Can you work these out from the model? Positions are in its coordinate system, mm. Face numbers are marked on the shaded views. Give positions to 0.01 mm unless a question says otherwise; leave off trailing zeros. Order: outer loops, then holes, each group sorted by start corner. A loop starts at its lowest first (then second) coordinate and runs counter-clockwise, first axis right, second up.
Item 1: I want a section at B-B, the plane y = 4.75. Write out the boundary of the cut face in (x, z), then the cut area to 3 significant figures.
Item 2: I want a section at D-D, the plane x = -0.75. Write out the boundary of the cut face in (y, z), then the cut area to 3 significant figures.
Item 3: If I drill on line 1 along Z through (x, y) = (-2, 3.9); line 2 along Z through (x, y) = (-2, 2.25); line 3 along X through (y, z) = (8, 4.5), over which ranges is the centre line in solid material (lowest first)?
Item 4: I want a section at C-C, the plane z = -14. Write out the boundary of the cut face in (x, y), then the cut area to 3 significant figures.
Item 5: I want a section at A-A, the plane z = -8. Write out the boundary of the cut face in (x, y).
Item 6: I'm going to push flat-ended pins straight in: pin 1 Ø5 at (x, z) = (-2, -8) entering from -Y; pin 2 Ø1.8 at (x, z) = (-2, -14) entering from -Y; pin 3 Ø3 at (x, z) = (-1, 3.5) entering from -Y. Where does each tip first touch, or does it pass through?
Item 7: If we mould it in two halves opening along X, with no side actions, what happens to the marked faces 1, 2, 3 and 4? For each: +X half, -X half, draft (parallel to the pull), parting line (faces both ways), or undercut.
Autodesk Inventor part; units mm, degrees
ref_plane "YZ Plane" through (0, 0, 0) normal (1, 0, 0) x (0, 1, 0)
ref_plane "XZ Plane" through (0, 0, 0) normal (0, 1, 0) x (-1, 0, 0)
ref_plane "XY Plane" through (0, 0, 0) normal (0, 0, 1) x (1, 0, 0)
sketch "Sketch1" plane through (0, 0, 0) normal (0, 1, 0) x (-1, 0, 0)
  line L0 (-6, 7) -> (10, 7)
  line L1 (10, 7) -> (10, -16)
  line L2 (10, -16) -> (-6, -16)
  line L3 (-6, -16) -> (-6, 7)
  point P0 (0, 0)
  point P1 (2, -8)
  point P2 (2, -14)
  point P3 (2, 4.5)
  dimension "d0" = 16
  dimension "d1" = 23
  dimension "d3" = 8
  dimension "d4" = 2
  dimension "d5" = 20.5
extrude "Extrusion1" add sketch "Sketch1" along normal blind 11.5
hole "Hole1" at (-2, 0, -8) direction (0, 1, 0) diameter 6 end through all
hole "Hole2" at (-2, 0, 4.5) direction (0, 1, 0) diameter 3 end through all
hole "Hole3" at (-2, 0, -14) direction (0, 1, 0) diameter 3 depth 6 tip angle 118
sketch "Sketch3" plane through (6, 0, 7) normal (1, 0, 0) x (0, 0, -1)
  arc A0 (5.6761, 2.9874) -> (5.6761, 5.0126) centre (8.5, 4) ccw
  line L0 (23, 0) -> (0, 0)
  line L1 (23, 0) -> (23, 11.5)
  line L2 (0, 0) -> (0, 11.5)
  line L3 (5.6761, 5.0126) -> (0, 5.0126)
  line L4 (5.6761, 2.9874) -> (0, 2.9874)
  line L5 (0, 5.0126) -> (0, 2.9874)
  point P0 (16, 0)
  point P1 (21, 5.75)
  dimension "d29" = 6
  dimension "d30" = 4
  dimension "d31" = 14.5
  dimension "d32" = 2
  dimension "d33" = 5.75
extrude "Extrusion2" cut sketch "Sketch3" against normal blind 20
hole "Hole4" at (6, 5.75, -14) direction (-1, 0, 0) diameter 3 end through all
thread "Thread1"
thread "Thread2"
thread "Thread3"
thread "Thread4"
properties part number "Chimera Heatblock" material "Aluminum 6061, Welded"
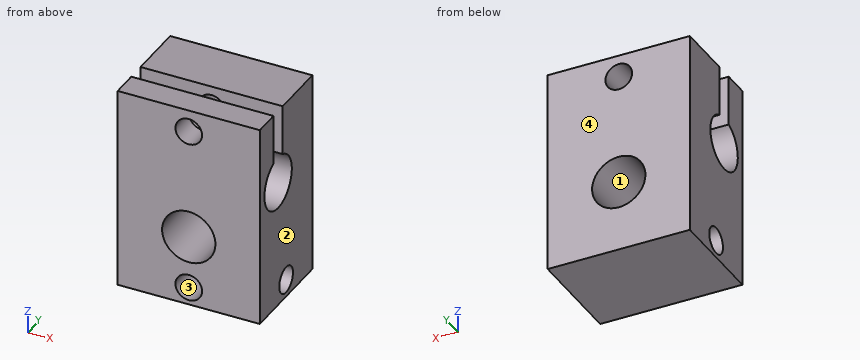
Results list:
1. outline: (-10, -16) - (6, -16) - (6, -15.12) - (-1, -15.12) arc R1.5 cw to (-3, -15.12) - (-10, -15.12) - close; (-10, -12.88) - (-3, -12.88) arc R1.5 cw to (-1, -12.88) - (6, -12.88) - (6, -4.4) - (-10, -4.4) - close; hole circle Ø6 at (-2, -8)
1. area: 120 mm2
2. outline: (0, -16) - (11.5, -16) - (11.5, -10.73) - (0, -10.73) - (0, -13.17) - (4.5, -13.17) arc R1.5 cw (long way) to (4.5, -14.83) - (0, -14.83) - close; (0, -5.27) - (11.5, -5.27) - (11.5, 3.67) - (5.01, 3.67) - (5.01, 1.32) arc R3 cw (long way) to (2.99, 1.32) - (2.99, 3.67) - (0, 3.67) - close; (0, 5.33) - (2.99, 5.33) - (2.99, 7) - (0, 7) - close; (5.01, 5.33) - (11.5, 5.33) - (11.5, 7) - (5.01, 7) - close
2. area: 132 mm2
3. line 1: z = -16 to -15.5, -12.5 to -11, -5 to -4.5
3. line 2: z = -16 to -15.5, -12.5 to -11, -5 to -3.94, 0.94 to 3, 6 to 7
3. line 3: x = -10 to -3.5, -0.5 to 6
4. outline: (-10, 0) - (-3.5, 0) - (-3.5, 4.25) - (-10, 4.25) - close; (-10, 7.25) - (6, 7.25) - (6, 11.5) - (-10, 11.5) - close; (-0.5, 0) - (6, 0) - (6, 4.25) - (-0.5, 4.25) - close
4. area: 123 mm2
5. outline: (-10, 0) - (-5, 0) - (-5, 11.5) - (-10, 11.5) - close; (1, 0) - (6, 0) - (6, 11.5) - (1, 11.5) - close
6. pin 1: passes through
6. pin 2: stops at y = 6.95
6. pin 3: stops at y = 0
7. face 1: undercut
7. face 2: +X half
7. face 3: undercut
7. face 4: draft
